Read the model definition and answer for the solid it produces. Units are mm, in the model's axes. Face numbers are marked on the shaded views. A direction names the side the tool comes from. Coordinates: 2 decimals unless noted, no trailing zeros. Loops run counter-clockwise (first coordinate to the right, second up) from the corner with the lowest first, then second, coordinate; pieces in that order, holes last. Notation, with made-up numbers: (14, 74) -> (64, 74) arc R29 cw to (64, 113) -> close; hole circle Ø5 at (63.5, 19). An arc over 180 degrees is marked (long way). Answer as a JSON object with one key per item and string values. Group by question number.
1) Section C-C, the plane y = -0.95 is taken. Give the vertices of the cut face in (x, z), plus the area to 3 significant figures.
2) Determine the mould class of the marked faces 1, 2 and 3 for opening direction X: released by +X, released by -X, zero draft, split by the parting line, or undercut.
3) Section B-B, the plane x = 0 is taken. Give the vertices of the cut face in (y, z), plus the area to 3 significant figures.
4) Flat-ended cylindrical pins translate along their axes: P1, Ø1.5, axis at x = -3, y = 2.5, coming from the -Z side; P2, Ø1.5, axis at x = 1, y = 3.5, coming from the -Z side. Find the tip coordinate at first contact, or state that the pin passes through.
5) Section D-D, the plane z = -4 is taken. Give the vertices of the cut face in (x, y), plus the area to 3 significant figures.
6) Which of the six approach directions +Z, -Z, +X, -X, +Y, -Y give full straight-line access (tool end or side, diameter ignored) to the marked faces 4 and 5?
7) Section A-A, the plane z = 2.75 is taken. Give the vertices of the cut face in (x, y).
8) Consider probe 1 along X at (y, z) = (1.2, 3.5); probe 2 along Z at (x, y) = (-0.5, 2.85); probe 3 along Y at (x, z) = (-1.5, 3.25). Determine where each line is inside the solid, lowest interval first. Write a range as [from, to].
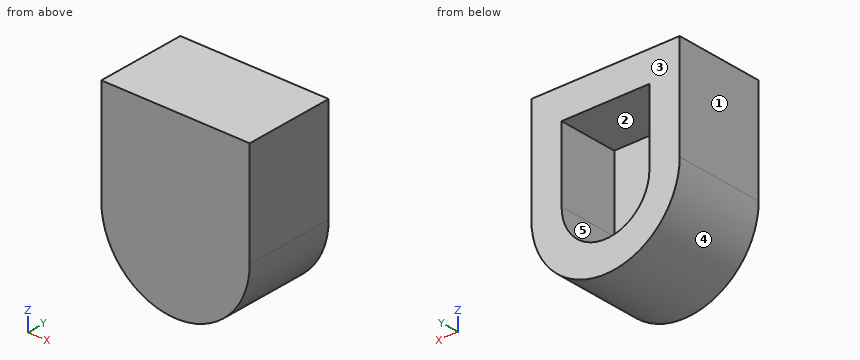
from build123d import *

# Parameters (mm, degrees)
BOSS_EXTRUDE1_DEPTH = 4
BOSS_EXTRUDE2_START = -2
BOSS_EXTRUDE2_DEPTH = 2


with BuildPart() as part:
    # Sketch1 → Boss-Extrude1 (new body)
    with BuildSketch(Plane(origin=(0, 0, 0), x_dir=(1, 0, 0), z_dir=(0, 1, 0))):
        with BuildLine():
            Line((-4.9, 0), (-2.9, 0))
            ThreePointArc((-2.9, 0), (0, 2.9), (2.9, 0))
            Line((2.9, 0), (4.9, 0))
            ThreePointArc((4.9, 0), (0, 4.9), (-4.9, 0))
        make_face()
        with BuildLine():
            Line((-2.9, -3.949683532), (-2.9, 0))
            Line((-2.9, 0), (-4.9, 0))
            ThreePointArc((-4.9, 0), (-4.371498599, -2.213594362), (-2.9, -3.949683532))
        make_face()
        with BuildLine():
            Line((-2.9, -4.9), (-2.9, -3.949683532))
            ThreePointArc((-2.9, -3.949683532), (-4.371498599, -2.213594362), (-4.9, 0))
            Line((-4.9, 0), (-4.9, -6.9))
            Line((-4.9, -6.9), (4.9, -6.9))
            Line((4.9, -6.9), (4.9, 0))
            ThreePointArc((4.9, 0), (4.371498599, -2.213594362), (2.9, -3.949683532))
            Line((2.9, -3.949683532), (2.9, -4.9))
            Line((2.9, -4.9), (2.3e-08, -4.9))
            Line((2.3e-08, -4.9), (-2.9, -4.9))
        make_face()
        with BuildLine():
            Line((4.9, 0), (2.9, 0))
            Line((2.9, 0), (2.9, -3.949683532))
            ThreePointArc((2.9, -3.949683532), (4.371498599, -2.213594362), (4.9, 0))
        make_face()
    extrude(amount=BOSS_EXTRUDE1_DEPTH)

    # Sketch1_3 → Boss-Extrude2 (add)
    with BuildSketch(Plane(origin=(0, 0, 0), x_dir=(1, 0, 0), z_dir=(0, 1, 0)).offset(BOSS_EXTRUDE2_START)):
        with BuildLine():
            Line((-2.9, -4.9), (-2.9, -3.949683532))
            ThreePointArc((-2.9, -3.949683532), (-4.371498599, -2.213594362), (-4.9, 0))
            Line((-4.9, 0), (-4.9, -6.9))
            Line((-4.9, -6.9), (4.9, -6.9))
            Line((4.9, -6.9), (4.9, 0))
            ThreePointArc((4.9, 0), (4.371498599, -2.213594362), (2.9, -3.949683532))
            Line((2.9, -3.949683532), (2.9, -4.9))
            Line((2.9, -4.9), (2.3e-08, -4.9))
            Line((2.3e-08, -4.9), (-2.9, -4.9))
        make_face()
        with BuildLine():
            ThreePointArc((2.3e-08, -4.9), (-1.525868708, -4.656363891), (-2.9, -3.949683532))
            Line((-2.9, -3.949683532), (-2.9, -4.9))
            Line((-2.9, -4.9), (2.3e-08, -4.9))
        make_face()
        with BuildLine():
            Line((2.9, -4.9), (2.9, -3.949683532))
            ThreePointArc((2.9, -3.949683532), (1.52586873, -4.656363884), (2.3e-08, -4.9))
            Line((2.3e-08, -4.9), (2.9, -4.9))
        make_face()
        with BuildLine():
            ThreePointArc((2.9, 0), (0, -2.9), (-2.9, 0))
            Line((-2.9, 0), (-2.9, -3.949683532))
            ThreePointArc((-2.9, -3.949683532), (-1.525868708, -4.656363891), (2.3e-08, -4.9))
            ThreePointArc((2.3e-08, -4.9), (1.52586873, -4.656363884), (2.9, -3.949683532))
            Line((2.9, -3.949683532), (2.9, 0))
        make_face()
        with BuildLine():
            Line((4.9, 0), (2.9, 0))
            Line((2.9, 0), (2.9, -3.949683532))
            ThreePointArc((2.9, -3.949683532), (4.371498599, -2.213594362), (4.9, 0))
        make_face()
        with BuildLine():
            Line((-2.9, -3.949683532), (-2.9, 0))
            Line((-2.9, 0), (-4.9, 0))
            ThreePointArc((-4.9, 0), (-4.371498599, -2.213594362), (-2.9, -3.949683532))
        make_face()
        with BuildLine():
            Line((-4.9, 0), (-2.9, 0))
            ThreePointArc((-2.9, 0), (0, 2.9), (2.9, 0))
            Line((2.9, 0), (4.9, 0))
            ThreePointArc((4.9, 0), (0, 4.9), (-4.9, 0))
        make_face()
        with BuildLine():
            ThreePointArc((2.9, 0), (0, 2.9), (-2.9, 0))
            Line((-2.9, 0), (2.9, 0))
        make_face()
        with BuildLine():
            Line((2.9, 0), (-2.9, 0))
            ThreePointArc((-2.9, 0), (0, -2.9), (2.9, 0))
        make_face()
    extrude(amount=BOSS_EXTRUDE2_DEPTH)


solid = part.part
Determined:
{
 "1": {"outline": "(-4.9, 0) arc R4.9 ccw to (4.9, 0) -> (4.9, 6.9) -> (-4.9, 6.9) -> close", "area": "105 mm²"},
 "2": {"face 1": "released by -X", "face 2": "undercut", "face 3": "zero draft"},
 "3": {"outline": "(-2, -4.9) -> (4, -4.9) -> (4, -2.9) -> (0, -2.9) -> (0, 4.9) -> (4, 4.9) -> (4, 6.9) -> (-2, 6.9) -> close", "area": "39.6 mm²"},
 "4": {"P1": "z = -4.35", "P2": "z = -4.89"},
 "5": {"outline": "(-2.83, -2) -> (2.83, -2) -> (2.83, 4) -> (-2.83, 4) -> close", "area": "34.0 mm²"},
 "6": {"face 4": "-Z, +Y, -Y", "face 5": "+Y"},
 "7": {"outline": "(-4.9, -2) -> (4.9, -2) -> (4.9, 4) -> (2.9, 4) -> (2.9, 0) -> (-2.9, 0) -> (-2.9, 4) -> (-4.9, 4) -> close"},
 "8": {"probe 1": "[-4.9, -2.9], [2.9, 4.9]", "probe 2": "[-4.87, -2.86], [4.9, 6.9]", "probe 3": "[-2, 0]"}
}
